from build123d import *

# Parameters (mm, degrees)
F0_W      = 65
F0_H      = 105
F2_DEPTH  = 5
F3_DEPTH  = 35
F4_W      = 5
F4_H      = 5
F5_DEPTH  = 5
F6_W      = 5
F6_H      = 5
F7_DEPTH  = 5
F8_W      = 5
F8_H      = 10
F9_DEPTH  = 30
F11_W     = 10
F11_H     = 5
F12_DEPTH = 10
F10_W     = 10
F10_H     = 5
F13_DEPTH = 10
F14_DEPTH = 5
F15_DEPTH = 5
F16_W     = 20
F16_H     = 5
F17_DEPTH = 5
F18_W     = 35
F18_H     = 5
F19_DEPTH = 15
F21_W     = 29
F21_H     = 5
F22_DEPTH = 25
F20_W     = 29
F20_H     = 5
F23_DEPTH = 25
F24_R     = 2.49999
F25_R     = 4.99999


# Not quite as in the source:
# - a fillet or chamfer is up to 0.001 mm smaller than in the source, because OpenCascade refuses the exact size


with BuildPart() as f2:
    # F0 (on Top) → F2 (new body)
    with BuildSketch(Plane.XY):
        Rectangle(F0_W, F0_H)
    extrude(amount=F2_DEPTH)

    # F1 (on face) → F3 (join)
    with BuildSketch(Plane.XY):
        Polygon((-22.5, 52.5), (-27.5, 52.5), (-32.5, 52.5), (-32.5, 47.5), (-32.5, 42.5), (-27.5, 42.5), (-27.5, 47.5), (-22.5, 47.5), align=None)
        Polygon((27.5, 52.5), (22.5, 52.5), (22.5, 47.5), (27.5, 47.5), (27.5, 42.5), (32.5, 42.5), (32.5, 52.5), align=None)
    extrude(amount=F3_DEPTH)

    # F4 (on face) → F5 (join)
    with BuildSketch(Plane(origin=(27.5, 0, 0), x_dir=(0, -1, 0), z_dir=(-1, 0, 0))):
        with Locations((-45, 32.5)):
            Rectangle(F4_W, F4_H)
    extrude(amount=F5_DEPTH)

    # F6 (on face) → F7 (join)
    with BuildSketch(Plane.YZ.offset(-27.5)):
        with Locations((45, 32.5)):
            Rectangle(F6_W, F6_H)
    extrude(amount=F7_DEPTH)

    # F8 (on face) → F9 (join)
    with BuildSketch(Plane.XY.offset(5)):
        with Locations((30, -32.5)):
            Rectangle(F8_W, F8_H)
        with Locations((-30, -32.5)):
            Rectangle(F8_W, F8_H)
    extrude(amount=F9_DEPTH)

    # F11 (on face) → F12 (join)
    with BuildSketch(Plane(origin=(27.5, 0, 0), x_dir=(0, -1, 0), z_dir=(-1, 0, 0))):
        with Locations((32.5, 32.5)):
            Rectangle(F11_W, F11_H)
    extrude(amount=F12_DEPTH)

    # F10 (on face) → F13 (join)
    with BuildSketch(Plane.YZ.offset(-27.5)):
        with Locations((-32.5, 32.5)):
            Rectangle(F10_W, F10_H)
    extrude(amount=F13_DEPTH)

    # F14 (add): a face of the model
    f14_faces = [f2.faces().sort_by_distance(p)[0] for p in [
        (22.5, 49.2857142857, 21.7857142857),
    ]]
    extrude(f14_faces, amount=F14_DEPTH)

    # F15 (add): a face of the model
    f15_faces = [f2.faces().sort_by_distance(p)[0] for p in [
        (-22.5, 49.2857142857, 21.7857142857),
    ]]
    extrude(f15_faces, amount=F15_DEPTH)

    # F16 (on face) → F17 (join)
    with BuildSketch(Plane.XY.offset(5)):
        with Locations((0, -50)):
            Rectangle(F16_W, F16_H)
    extrude(amount=F17_DEPTH)

    # F18 (on face) → F19 (join)
    with BuildSketch(Plane(origin=(0, 0, 0), x_dir=(1, 0, 0), z_dir=(0, 0, -1))):
        with Locations((0, 50)):
            Rectangle(F18_W, F18_H)
        with Locations((0, -50)):
            Rectangle(F18_W, F18_H)
    extrude(amount=F19_DEPTH)

    # F21 (on face) → F22 (cut)
    with BuildSketch(Plane.XZ.offset(-47.5)):
        with Locations((0, -8.5)):
            Rectangle(F21_W, F21_H)
    extrude(amount=-F22_DEPTH, mode=Mode.SUBTRACT)

    # F20 (on face) → F23 (cut)
    with BuildSketch(Plane(origin=(0, -47.5, 0), x_dir=(-1, 0, 0), z_dir=(0, 1, 0))):
        with Locations((0, -8.5)):
            Rectangle(F20_W, F20_H)
    extrude(amount=-F23_DEPTH, mode=Mode.SUBTRACT)

    # F24 (radius 2.5 in the source; OpenCascade refuses exactly that, so slightly less here)
    f24_edges = [f2.edges().sort_by_distance(p)[0] for p in [
        (0, 52.5, -15),
        (0, 47.5, -15),
        (0, -52.5, -15),
        (0, -47.5, -15),
    ]]
    fillet(f24_edges, radius=F24_R)

    # F25 (radius 5 in the source; OpenCascade refuses exactly that, so slightly less here)
    f25_edges = [f2.edges().sort_by_distance(p)[0] for p in [
        (-32.5, -32.5, 35),
        (32.5, -32.5, 35),
        (17.5, -32.5, 35),
        (-17.5, -32.5, 35),
        (-25, 52.5, 35),
        (25, 52.5, 35),
        (32.5, 47.5, 35),
        (25, 42.5, 35),
        (17.5, 47.5, 35),
        (-25, 42.5, 35),
        (-17.5, 47.5, 35),
        (-32.5, 47.5, 35),
        (-25, -37.5, 35),
        (-25, -27.5, 35),
        (25, -37.5, 35),
        (25, -27.5, 35),
        (0, -52.5, 10),
    ]]
    fillet(f25_edges, radius=F25_R)


solid = f2.part
Source: CAD feature listing. Evaluate the final solid. Frame: model axes, mm. A direction names the side the tool comes from. Round coordinates to 2 decimals unless told otherwise and drop trailing zeros. Write each loop counter-clockwise with the first axis right and the second up, starting at its lowest first coordinate (ties: lowest second). Pieces come first, ordered by that corner, then holes. Notation, with made-up numbers: M -7.75,84.5 L 21.25,84.5 A19 cw 21.25,113.5 Z; hole C 57.5,-6.75 d4. An arc over 180 degrees is marked long. One line per item, written item: value. Start each with the question number.
Item 1: Section query B-B (z = 25). Return the cut outline in (x, y), plus the area to 3 significant figures.
Item 2: Section query A-A (x = 1.5). State how many separate pieces and enclosed holes the cut face has, plus the area to 3 significant figures.
Item 3: Set-up query: faces 4 (the flat face through (17.5, 50, -7)), 5 (the flat face through (-27.5, -33, 17)), 6 (the cylindrical face through (25.105, -28.436, 32.913)), 7 (the cylindrical face through (18.436, -32.57, 32.913)). Return all of +Z, -Z, +X, -X, +Y, -Y with unobstructed straight access to the full face (end or side cutting, diameter ignored); none if empty.
Item 4: Mould query, pull axis Z, two halves, no side actions, for faces 1 (the flat face through (23, 47.5, 17)), 2 (the flat face through (0, -52.5, -2)), 3 (the cylindrical face through (0, -48, -14)). Classes: pulls with the +Z half, pulls with the -Z half, needs draft (parallel to the pull), parting line crosses it, or undercut.
Item 5: Pin query (flat end, axial travel): pin 1 (1.5 mm diameter, centred on x = -25.5, z = -1, fed in from +Y); pin 2 (5.5 mm diameter, centred on x = -3.5, y = -50.5, fed in from +Z); pin 3 (8 mm diameter, centred on x = 1, y = -33.5, fed in from -Z); pin 4 (5.5 mm diameter, centred on x = -4, y = 51, fed in from +Z). Return the tip coordinate at first contact, or that it passes through.
Item 6: Ray query, L1, parallel to Z at x = 14, y = 39; L2, parallel to Z at x = -21, y = -35; L3, parallel to Y at x = 20.5, z = 8.5. Return the intervals inside material, ascending. Write a range as from..to.
Item 7: Section query D-D (z = -7.5). Return the cut outline in (x, y), plus the area to 3 significant figures.
Result set:
1. outline: M -32.5,-37.5 L -27.5,-37.5 L -27.5,-27.5 L -32.5,-27.5 Z; M -32.5,42.5 L -27.5,42.5 L -27.5,47.5 L -17.5,47.5 L -17.5,52.5 L -32.5,52.5 Z; M 17.5,47.5 L 27.5,47.5 L 27.5,42.5 L 32.5,42.5 L 32.5,52.5 L 17.5,52.5 Z; M 27.5,-37.5 L 32.5,-37.5 L 32.5,-27.5 L 27.5,-27.5 Z
1. area: 300 mm²
2. separate pieces: 3
2. enclosed holes: 0
2. area: 639 mm²
3. face 4: -Z, +X, +Y, -Y
3. face 5: -Y
3. face 6: +Z, +X, -X
3. face 7: +Z, +Y, -Y
4. face 1: undercut
4. face 2: needs draft
4. face 3: pulls with the -Z half
5. pin 1: passes through
5. pin 2: stops at z = 9.99
5. pin 3: stops at z = 0
5. pin 4: stops at z = 5
6. L1: z = 0..5
6. L2: z = 0..5, 30..34.33
6. L3: y = 47.5..52.5
7. outline: M -17.5,-52.5 L -14.5,-52.5 L -14.5,-47.5 L -17.5,-47.5 Z; M -17.5,47.5 L -14.5,47.5 L -14.5,52.5 L -17.5,52.5 Z; M 14.5,-52.5 L 17.5,-52.5 L 17.5,-47.5 L 14.5,-47.5 Z; M 14.5,47.5 L 17.5,47.5 L 17.5,52.5 L 14.5,52.5 Z
7. area: 60.0 mm²
